Autodesk Inventor part; units mm, degrees
ref_plane "YZ Plane" through (0, 0, 0) normal (1, 0, 0) x (0, 1, 0)
ref_plane "XZ Plane" through (0, 0, 0) normal (0, 1, 0) x (-1, 0, 0)
ref_plane "XY Plane" through (0, 0, 0) normal (0, 0, 1) x (1, 0, 0)
sketch "Sketch1" plane through (0, 0, 0) normal (0, 0, 1) x (1, 0, 0)
  line L0 (-26.5, 6.25) -> (26.5, 6.25)
  line L1 (26.5, 6.25) -> (26.5, -6.25)
  line L2 (26.5, -6.25) -> (-26.5, -6.25)
  line L3 (-26.5, -6.25) -> (-26.5, 6.25)
  line L4 (-26.5, 6.25) -> (26.5, -6.25) construction
  line L5 (26.5, 6.25) -> (-26.5, -6.25) construction
  line L6 (-26.5, 0) -> (26.5, 0) construction
  circle A0 centre (-23.5, 0) radius 1.25
  circle A1 centre (-23.5, 0) radius 2.8868 construction
  line L7 (-22.0566, -2.5) -> (-24.9434, 2.5) construction
  line L8 (-26.3868, 0) -> (-20.6132, 0) construction
  line L9 (-22.0566, 2.5) -> (-24.9434, -2.5) construction
  line L10 (-22.0566, 2.5) -> (-24.9434, 2.5)
  line L11 (-24.9434, 2.5) -> (-26.3868, 0)
  line L12 (-24.9434, -2.5) -> (-26.3868, 0)
  line L13 (-22.0566, -2.5) -> (-24.9434, -2.5)
  line L14 (-20.6132, 0) -> (-22.0566, 2.5)
  line L15 (-20.6132, 0) -> (-22.0566, -2.5)
  line L16 (0, 6.25) -> (0, -6.25) construction
  circle A2 centre (23.5, 0) radius 1.25
  line L17 (22.0566, 2.5) -> (24.9434, 2.5)
  line L18 (24.9434, 2.5) -> (26.3868, 0)
  line L19 (24.9434, -2.5) -> (26.3868, 0)
  line L20 (22.0566, -2.5) -> (24.9434, -2.5)
  line L21 (20.6132, 0) -> (22.0566, 2.5)
  line L22 (20.6132, 0) -> (22.0566, -2.5)
  line L23 (-18, 4.5) -> (18, 4.5)
  line L24 (-18, 4.5) -> (-19.5, 2.3)
  line L25 (-19.5, 2.3) -> (-19, -2.3)
  line L26 (-19, -2.3) -> (-17, -4.5)
  line L27 (-17, -4.5) -> (17, -4.5)
  line L28 (17, -4.5) -> (19, -2.3)
  line L29 (19, -2.3) -> (19.5, 2.3)
  line L30 (19.5, 2.3) -> (18, 4.5)
  point P0 (0, 0)
  point P1 (0, 4.5)
  point P2 (0, -4.5)
  dimension "d0" = 53
  dimension "d1" = 12.5
  dimension "d2" = 2.5
  dimension "d4" = 60
  dimension "d5" = 60
  dimension "d6" = 5
  dimension "d7" = 47
  dimension "d8" = 39
  dimension "d9" = 34
  dimension "d10" = 36
  dimension "d11" = 38
  dimension "d12" = 9
  dimension "d13" = 2.2
  dimension "d14" = 2.2
extrude "Extrusion1" add sketch "Sketch1" along normal blind 5 contours L14 L15 L13 L12 L11 L10 | L17 L18 L19 L20 L22 L21
extrude "Extrusion2" add sketch "Sketch1" along normal blind 6 contours L23 L30 L29 L28 L27 L26 L25 L24
extrude "Extrusion3" add sketch "Sketch1" against normal blind 12 contours L0 L1 L2 L3 | A0 | L14 L15 L13 L12 L11 L10 | A2 | L17 L18 L19 L20 L22 L21 | L23 L30 L29 L28 L27 L26 L25 L24
sketch "Sketch2" plane through (0, 0, -12) normal (0, 0, -1) x (-1, 0, 0)
  line L0 (26.5, 6.25) -> (-26.5, 6.25)
  line L1 (-26.5, 6.25) -> (-26.5, -6.25)
  line L2 (-26.5, -6.25) -> (26.5, -6.25)
  line L3 (26.5, -6.25) -> (26.5, 6.25)
  line L4 (-26.5, 6.25) -> (-26.5, -6.25)
  line L5 (-26.5, -3.25) -> (-20, -3.25)
  line L6 (-20, -3.25) -> (-20, 4.25)
  line L7 (-20, 4.25) -> (20, 4.25)
  line L8 (20, 4.25) -> (20, -3.25)
  line L9 (20, -3.25) -> (26.5, -3.25)
  line L10 (0, 6.25) -> (0, -6.25) construction
  line L11 (-26.5, -3.25) -> (-26.5, 6.25)
  line L12 (26.5, 6.25) -> (-26.5, 6.25)
  line L13 (-26.5, 6.25) -> (26.5, 6.25)
  line L14 (26.5, 6.25) -> (26.5, -3.25)
  point P0 (0, 0)
  dimension "d21" = 40
  dimension "d22" = 2
  dimension "d23" = 3
extrude "Extrusion4" cut sketch "Sketch2" against normal blind 9 contours L3 L9 L8 L7 L6 L5 L1 L0
sketch "Sketch3" plane through (0, 0, 0) normal (0, 1, 0) x (-1, 0, 0)
  line L0 (26.5, -3) -> (26.5, -12)
  line L1 (26.5, -12) -> (20, -12)
  line L2 (20, -12) -> (20, -3)
  arc A0 (23.25, -3.75) -> (21.25, -5.75) centre (23.25, -5.75) ccw
  arc A1 (23.25, -11.25) -> (25.25, -9.25) centre (23.25, -9.25) ccw
  line L3 (23.25, -3.75) -> (23.25, -11.25) construction
  line L4 (25.25, -5.75) -> (25.25, -9.25)
  line L5 (21.25, -9.25) -> (21.25, -5.75)
  line L6 (25.25, -7.5) -> (21.25, -7.5) construction
  line L7 (26.5, -3) -> (20, -3)
  arc A2 (21.25, -9.25) -> (23.25, -11.25) centre (23.25, -9.25) ccw
  arc A3 (25.25, -9.25) -> (21.25, -9.25) centre (23.25, -9.25) ccw construction
  arc A4 (25.25, -5.75) -> (23.25, -3.75) centre (23.25, -5.75) ccw
  arc A5 (21.25, -5.75) -> (25.25, -5.75) centre (23.25, -5.75) ccw construction
  line L8 (0, 0) -> (0, -12) construction
  arc A6 (-21.25, -5.75) -> (-23.25, -3.75) centre (-23.25, -5.75) ccw
  arc A7 (-25.25, -9.25) -> (-23.25, -11.25) centre (-23.25, -9.25) ccw
  line L9 (-25.25, -5.75) -> (-25.25, -9.25)
  line L10 (-21.25, -9.25) -> (-21.25, -5.75)
  arc A8 (-23.25, -11.25) -> (-21.25, -9.25) centre (-23.25, -9.25) ccw
  arc A9 (-23.25, -3.75) -> (-25.25, -5.75) centre (-23.25, -5.75) ccw
  dimension "d26" = 4
  dimension "d27" = 7.5
  dimension "d28" = 9
  dimension "d29" = 4.5
  dimension "d30" = 6.5
  dimension "d31" = 3.25
extrude "Extrusion5" cut sketch "Sketch3" against normal through all contours A4 L4 A1 A2 L5 A0 | L10 A8 A7 L9 A9 A6
sketch "Sketch4" plane through (0, 0, 6) normal (0, 0, 1) x (1, 0, 0)
  line L0 (-16.2, 1.8249) -> (16.2, 1.8249) construction
  circle A0 centre (-16.2, 1.8249) radius 0.5
  circle A1 centre (-13.5, 1.8249) radius 0.5
  circle A2 centre (-10.8, 1.8249) radius 0.5
  circle A3 centre (-8.1, 1.8249) radius 0.5
  circle A4 centre (-5.4, 1.8249) radius 0.5
  circle A5 centre (-2.7, 1.8249) radius 0.5
  circle A6 centre (0, 1.8249) radius 0.5
  circle A7 centre (2.7, 1.8249) radius 0.5
  circle A8 centre (5.4, 1.8249) radius 0.5
  circle A9 centre (8.1, 1.8249) radius 0.5
  circle A10 centre (10.8, 1.8249) radius 0.5
  circle A11 centre (13.5, 1.8249) radius 0.5
  circle A12 centre (16.2, 1.8249) radius 0.5
  line L1 (-14.85, -1.8249) -> (14.85, -1.8249) construction
  circle A13 centre (-14.85, -1.8249) radius 0.5
  circle A14 centre (-12.15, -1.8249) radius 0.5
  circle A15 centre (-9.45, -1.8249) radius 0.5
  circle A16 centre (-6.75, -1.8249) radius 0.5
  circle A17 centre (-4.05, -1.8249) radius 0.5
  circle A18 centre (-1.35, -1.8249) radius 0.5
  circle A19 centre (1.35, -1.8249) radius 0.5
  circle A20 centre (4.05, -1.8249) radius 0.5
  circle A21 centre (6.75, -1.8249) radius 0.5
  circle A22 centre (9.45, -1.8249) radius 0.5
  circle A23 centre (12.15, -1.8249) radius 0.5
  circle A24 centre (14.85, -1.8249) radius 0.5
  line L2 (0, 1.8249) -> (0, -1.8249) construction
  line L3 (18, 4.5) -> (-18, 4.5) construction
  line L4 (-18, 4.5) -> (-19.5, 2.3) construction
  line L5 (-19.5, 2.3) -> (-19, -2.3) construction
  line L6 (-19, -2.3) -> (-17, -4.5) construction
  line L7 (-17, -4.5) -> (17, -4.5) construction
  line L8 (17, -4.5) -> (19, -2.3) construction
  line L9 (19, -2.3) -> (19.5, 2.3) construction
  line L10 (19.5, 2.3) -> (18, 4.5) construction
  line L11 (-17.7357, 4) -> (17.7357, 4)
  line L12 (17.7357, 4) -> (18.983, 2.1707)
  line L13 (18.983, 2.1707) -> (18.5205, -2.0841)
  line L14 (18.5205, -2.0841) -> (16.7788, -4)
  line L15 (16.7788, -4) -> (-16.7788, -4)
  line L16 (-16.7788, -4) -> (-18.5205, -2.0841)
  line L17 (-18.5205, -2.0841) -> (-18.983, 2.1707)
  line L18 (-18.983, 2.1707) -> (-17.7357, 4)
  point P0 (0, 0)
  point P1 (0, 0)
  dimension "d34" = 1
  dimension "d37" = 2.7
  dimension "d44" = 2.7
  dimension "d49" = 0.5
extrude "Extrusion6" cut sketch "Sketch4" against normal up to surface (6 mm away)
fillet "Fillet1" radius 1 4 edges at (-26.5, 6.25, -1.5) (26.5, 6.25, -1.5) (20, 4.25, -7.5) (-20, 4.25, -7.5)
equation "\"d5\" = d4"
equation "\"d14\" = d13"
equation "\"d29\" = 0.5 * d28"
equation "\"d31\" = 0.5 * d30"
equation "\"d44\" = d37"
properties part number "db25-connector-pcb"
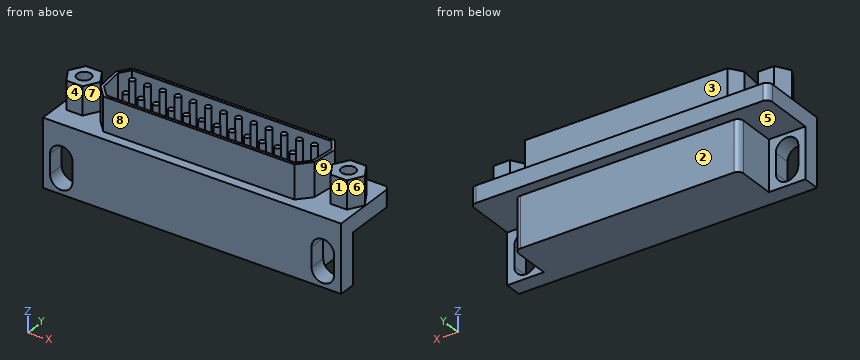
Design review of the part built by this model. Coordinates are the model's own, in mm. Face numbers are marked on the shaded views. A direction names the side the tool comes from. Round coordinates to 2 decimals unless told otherwise and drop trailing zeros. Order: outer loops, then holes, each group sorted by start corner. A loop starts at its lowest first (then second) coordinate and runs counter-clockwise, first axis right, second up. Notation, with made-up numbers: (-7, 10.25) - (37, 10.25) arc R24 ccw to (37, 37.25) - close; hole circle Ø10 at (73, -27.5). An arc over 180 degrees is marked (long way). Return JSON: item names as keys, results as strings.
Q1. Machinability: for the marked faces 1, 2, 3, 4 and 5, which of the approach directions +Z, -Z, +X, -X, +Y, -Y give a long, thin tool a straight path to every point of the face, cutting with its end or side? Answer none if there is none.
Computed values:
{"face 1": "+Z, +X, -Y", "face 2": "-Z, +X, -X, +Y", "face 3": "+Z, +X, -X, +Y", "face 4": "+Z, -X, -Y", "face 5": "-Z, +Y"}
Q2. Consider section B-B on z = -8.25. Write out the cut boundary in (x, y).
Computed values:
{"outline": "(-26.5, -6.25) - (-25.25, -6.25) - (-25.25, -3.25) - (-26.5, -3.25) - close; (-21.25, -6.25) - (21.25, -6.25) - (21.25, -3.25) - (20, -3.25) - (20, 3.25) arc R1 ccw to (19, 4.25) - (-19, 4.25) arc R1 ccw to (-20, 3.25) - (-20, -3.25) - (-21.25, -3.25) - close; (25.25, -6.25) - (26.5, -6.25) - (26.5, -3.25) - (25.25, -3.25) - close"}
Q3. For pin 1 Ø5 at (x, z) = (23, -9) entering from +Y; pin 2 Ø1.8 at (x, z) = (-0.5, 4.5) entering from +Y; pin 3 Ø5 at (y, z) = (2.5, -7.5) entering from +X, all flat-tipped, find the tip position at first contact; note any pin that passes through.
Computed values:
{"pin 1": "stops at y = -3.25", "pin 2": "stops at y = 4.5", "pin 3": "stops at x = 20"}
Q4. Wall thickness on L1, parallel to Y at x = 13.5, z = 2.5; L2, parallel to Y at x = 23.5, z = 2.9; L3, parallel to X at y = 3.25, z = -7.25: over which ranges is each line inside the solid? List them lowest first. Write a range as [from, to].
Computed values:
{"L1": "y = [-4.5, -4], [1.32, 2.32], [4, 4.5]", "L2": "y = [-2.5, -1.25], [1.25, 2.5]", "L3": "x = [-20, 20]"}
Q5. The part is to be moulded in two halves that separate along X. For the marked faces 6, 7, 8 and 9, say which applies: pulls with the +X half, pulls with the -X half, needs draft (parallel to the pull), parting line crosses it, or undercut.
Computed values:
{"face 6": "pulls with the +X half", "face 7": "undercut", "face 8": "needs draft", "face 9": "undercut"}
Q6. Consider section A-A on x = 2.7. Write out the cut boundary in (y, z), plus the area to 3 significant figures.
Computed values:
{"outline": "(-6.25, -12) - (4.25, -12) - (4.25, -3) - (6.25, -3) - (6.25, 0) - (4.5, 0) - (4.5, 6) - (4, 6) - (4, 0) - (2.32, 0) - (2.32, 6) - (1.32, 6) - (1.32, 0) - (-4, 0) - (-4, 6) - (-4.5, 6) - (-4.5, 0) - (-6.25, 0) - close", "area": "144 mm2"}
